Could you check a few things on this model? Use its own coordinates, in mm. Face numbers are marked on the shaded views. A direction names the side the tool comes from. Coordinates: 2 decimals unless noted, no trailing zeros. Order: outer loops, then holes, each group sorted by start corner. A loop starts at its lowest first (then second) coordinate and runs counter-clockwise, first axis right, second up. Notation, with made-up numbers: (40, 3.5) - (85, 3.5) arc R17 ccw to (85, 34.5) - close; hole circle Ø6 at (79, 73). An arc over 180 degrees is marked (long way). Answer as a JSON object with one key per item and string values. Group by question number.
(1) Which directions (+Z, -Z, +X, -X, +Y, -Y) give clear straight access to the entire face, cutting with the end or side of a thin tool? Please do the marked faces 1 and 2.
(2) Imagine slicing it at D-D, the plane x = -15.5. Write out the boundary of the cut face in (y, z).
(3) Imagine slicing it at A-A, the plane z = 1.6. Write out the boundary of the cut face in (x, y).
(4) Will these pins go through, and if not, where does the flat tip stop? P1, Ø10, axis at x = -59, y = 3, coming from the +Z side; P2, Ø1, axis at x = -67.5, z = -0.5, coming from the -Y side; P3, Ø4, axis at x = -10.5, y = 19.5, coming from the -Z side; P4, Ø0.7, axis at y = -52.5, z = 0, coming from the -X side.
(5) Imagine slicing it at B-B, the plane x = 0. Write out the boundary of the cut face in (y, z).
(6) Please list where these lines run through material, in increasing order: probe 1 along Y at (x, z) = (-0.5, 2.45); probe 2 along Y at (x, z) = (-13.5, -0.35); probe 3 along X at (y, z) = (-6.5, -0.65).
(7) Imagine slicing it at C-C, the plane y = -72. Write out the boundary of the cut face in (x, z), and give its area (3 significant figures).
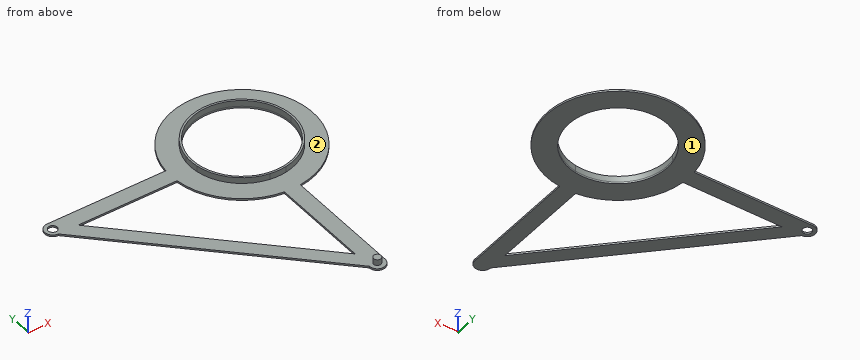
from build123d import *

# Parameters (mm, degrees)
F1_DEPTH = 0.9
F2_DEPTH = 3
F3_DEPTH = 3


with BuildPart() as f1:
    # F0 (on Top) → F1 (new body)
    with BuildSketch(Plane.XY):
        with BuildLine():
            Line((-35.5758344948, 4), (-95.5, 4))
            ThreePointArc((-95.5, 4), (-92.6715728753, 2.8284271247), (-91.5, 0))
            ThreePointArc((-91.5, 0), (-92.6715728753, -2.8284271247), (-95.5, -4))
            Line((-95.5, -4), (-85.6005050634, -4))
            Line((-85.6005050634, -4), (-35.5758344948, -4))
            ThreePointArc((-35.5758344948, -4), (-35.8, 0), (-35.5758344948, 4))
        make_face()
        with BuildLine():
            ThreePointArc((-95.5, 2.25), (-93.9090097423, 1.5909902577), (-93.25, 0))
            ThreePointArc((-93.25, 0), (-93.9090097423, -1.5909902577), (-95.5, -2.25))
            Line((-95.5, -2.25), (-95.5, -4))
            ThreePointArc((-95.5, -4), (-92.6715728753, -2.8284271247), (-91.5, 0))
            ThreePointArc((-91.5, 0), (-92.6715728753, 2.8284271247), (-95.5, 4))
            Line((-95.5, 4), (-95.5, 2.25))
        make_face()
        with BuildLine():
            ThreePointArc((-95.5, -2.25), (-97.75, 0), (-95.5, 2.25))
            Line((-95.5, 2.25), (-95.5, 4))
            ThreePointArc((-95.5, 4), (-99.5, 0), (-95.5, -4))
            Line((-95.5, -4), (-95.5, -2.25))
        make_face()
        Polygon((-85.6005050634, -4), (-95.5, -4), (-4, -95.5), (-4, -85.6005050634), align=None)
        with BuildLine():
            Line((-1.85, -95.5), (-4, -95.5))
            ThreePointArc((-4, -95.5), (0, -99.5), (4, -95.5))
            Line((4, -95.5), (1.85, -95.5))
            ThreePointArc((1.85, -95.5), (0, -97.35), (-1.85, -95.5))
        make_face()
        with BuildLine():
            ThreePointArc((4, -95.5), (0, -91.5), (-4, -95.5))
            Line((-4, -95.5), (-1.85, -95.5))
            ThreePointArc((-1.85, -95.5), (0, -93.65), (1.85, -95.5))
            Line((1.85, -95.5), (4, -95.5))
        make_face()
        with BuildLine():
            Line((1.85, -95.5), (-1.85, -95.5))
            ThreePointArc((-1.85, -95.5), (0, -97.35), (1.85, -95.5))
        make_face()
        with BuildLine():
            ThreePointArc((1.85, -95.5), (0, -93.65), (-1.85, -95.5))
            Line((-1.85, -95.5), (1.85, -95.5))
        make_face()
        with BuildLine():
            Line((-4, -85.6005050634), (-4, -95.5))
            ThreePointArc((-4, -95.5), (0, -91.5), (4, -95.5))
            Line((4, -95.5), (4, -35.5758344948))
            ThreePointArc((4, -35.5758344948), (0, -35.8), (-4, -35.5758344948))
            Line((-4, -35.5758344948), (-4, -85.6005050634))
        make_face()
        with BuildLine():
            Line((-25.4880364093, -4), (-35.5758344948, -4))
            ThreePointArc((-35.5758344948, -4), (-25.3144227665, -25.3144227665), (-4, -35.5758344948))
            Line((-4, -35.5758344948), (-4, -25.4880364093))
            ThreePointArc((-4, -25.4880364093), (-18.2433549546, -18.2433549546), (-25.4880364093, -4))
        make_face()
        with BuildLine():
            Line((-25.4880364093, 4), (-35.5758344948, 4))
            ThreePointArc((-35.5758344948, 4), (-35.8, 0), (-35.5758344948, -4))
            Line((-35.5758344948, -4), (-25.4880364093, -4))
            ThreePointArc((-25.4880364093, -4), (-25.8, 0), (-25.4880364093, 4))
        make_face()
        with BuildLine():
            ThreePointArc((35.8, 0), (2.0031381738, 35.7439146913), (-35.5758344948, 4))
            Line((-35.5758344948, 4), (-25.4880364093, 4))
            ThreePointArc((-25.4880364093, 4), (2.0060733587, 25.7218908652), (25.8, 0))
            ThreePointArc((25.8, 0), (19.6066315312, -16.7696153802), (4, -25.4880364093))
            Line((4, -25.4880364093), (4, -35.5758344948))
            ThreePointArc((4, -35.5758344948), (26.6911970507, -23.858331878), (35.8, 0))
        make_face()
        with BuildLine():
            ThreePointArc((-4, -35.5758344948), (0, -35.8), (4, -35.5758344948))
            Line((4, -35.5758344948), (4, -25.4880364093))
            ThreePointArc((4, -25.4880364093), (0, -25.8), (-4, -25.4880364093))
            Line((-4, -25.4880364093), (-4, -35.5758344948))
        make_face()
        with BuildLine():
            Line((-24.5158234616, -4), (-25.4880364093, -4))
            ThreePointArc((-25.4880364093, -4), (-18.2433549546, -18.2433549546), (-4, -25.4880364093))
            Line((-4, -25.4880364093), (-4, -24.5158234616))
            ThreePointArc((-4, -24.5158234616), (-17.5645324447, -17.5645324447), (-24.5158234616, -4))
        make_face()
        with BuildLine():
            Line((-24.5158234616, 4), (-25.4880364093, 4))
            ThreePointArc((-25.4880364093, 4), (-25.8, 0), (-25.4880364093, -4))
            Line((-25.4880364093, -4), (-24.5158234616, -4))
            ThreePointArc((-24.5158234616, -4), (-24.84, 0), (-24.5158234616, 4))
        make_face()
        with BuildLine():
            ThreePointArc((25.8, 0), (2.0060733587, 25.7218908652), (-25.4880364093, 4))
            Line((-25.4880364093, 4), (-24.5158234616, 4))
            ThreePointArc((-24.5158234616, 4), (2.0065574019, 24.7588232231), (24.84, 0))
            ThreePointArc((24.84, 0), (18.925982141, -16.0882814496), (4, -24.5158234616))
            Line((4, -24.5158234616), (4, -25.4880364093))
            ThreePointArc((4, -25.4880364093), (19.6066315312, -16.7696153802), (25.8, 0))
        make_face()
        with BuildLine():
            ThreePointArc((-4, -25.4880364093), (0, -25.8), (4, -25.4880364093))
            Line((4, -25.4880364093), (4, -24.5158234616))
            ThreePointArc((4, -24.5158234616), (0, -24.84), (-4, -24.5158234616))
            Line((-4, -24.5158234616), (-4, -25.4880364093))
        make_face()
    extrude(amount=-F1_DEPTH)

    # F0 (on Top) → F2 (join)
    with BuildSketch(Plane.XY):
        with BuildLine():
            ThreePointArc((25.8, 0), (2.0060733587, 25.7218908652), (-25.4880364093, 4))
            Line((-25.4880364093, 4), (-24.5158234616, 4))
            ThreePointArc((-24.5158234616, 4), (2.0065574019, 24.7588232231), (24.84, 0))
            ThreePointArc((24.84, 0), (18.925982141, -16.0882814496), (4, -24.5158234616))
            Line((4, -24.5158234616), (4, -25.4880364093))
            ThreePointArc((4, -25.4880364093), (19.6066315312, -16.7696153802), (25.8, 0))
        make_face()
        with BuildLine():
            Line((-24.5158234616, 4), (-25.4880364093, 4))
            ThreePointArc((-25.4880364093, 4), (-25.8, 0), (-25.4880364093, -4))
            Line((-25.4880364093, -4), (-24.5158234616, -4))
            ThreePointArc((-24.5158234616, -4), (-24.84, 0), (-24.5158234616, 4))
        make_face()
        with BuildLine():
            Line((-24.5158234616, -4), (-25.4880364093, -4))
            ThreePointArc((-25.4880364093, -4), (-18.2433549546, -18.2433549546), (-4, -25.4880364093))
            Line((-4, -25.4880364093), (-4, -24.5158234616))
            ThreePointArc((-4, -24.5158234616), (-17.5645324447, -17.5645324447), (-24.5158234616, -4))
        make_face()
        with BuildLine():
            ThreePointArc((-4, -25.4880364093), (0, -25.8), (4, -25.4880364093))
            Line((4, -25.4880364093), (4, -24.5158234616))
            ThreePointArc((4, -24.5158234616), (0, -24.84), (-4, -24.5158234616))
            Line((-4, -24.5158234616), (-4, -25.4880364093))
        make_face()
    extrude(amount=F2_DEPTH)

    # F0 (on Top) → F3 (join)
    with BuildSketch(Plane.XY):
        with BuildLine():
            ThreePointArc((1.85, -95.5), (0, -93.65), (-1.85, -95.5))
            Line((-1.85, -95.5), (1.85, -95.5))
        make_face()
        with BuildLine():
            Line((1.85, -95.5), (-1.85, -95.5))
            ThreePointArc((-1.85, -95.5), (0, -97.35), (1.85, -95.5))
        make_face()
    extrude(amount=F3_DEPTH)


solid = f1.part
Result set:
{
 "1": {"face 1": "-Z, +X, -X, +Y, -Y", "face 2": "+Z"},
 "2": {"outline": "(-84, -0.9) - (-74.1, -0.9) - (-74.1, 0) - (-84, 0) - close; (-32.27, -0.9) - (-19.41, -0.9) - (-19.41, 3) - (-20.62, 3) - (-20.62, 0) - (-32.27, 0) - close; (19.41, -0.9) - (32.27, -0.9) - (32.27, 0) - (20.62, 0) - (20.62, 3) - (19.41, 3) - close"},
 "3": {"outline": "circle Ø51.6 at (0, 0); circle Ø3.7 at (0, -95.5); hole circle Ø49.68 at (0, 0)"},
 "4": {"P1": "stops at z = 0", "P2": "stops at y = -32.5", "P3": "passes through", "P4": "stops at x = -47.35"},
 "5": {"outline": "(-99.5, -0.9) - (-24.84, -0.9) - (-24.84, 3) - (-25.8, 3) - (-25.8, 0) - (-93.65, 0) - (-93.65, 3) - (-97.35, 3) - (-97.35, 0) - (-99.5, 0) - close; (24.84, -0.9) - (35.8, -0.9) - (35.8, 0) - (25.8, 0) - (25.8, 3) - (24.84, 3) - close"},
 "6": {"probe 1": "y = -97.28 to -93.72, -25.8 to -24.83, 24.83 to 25.8", "probe 2": "y = -86 to -76.1, -33.16 to -20.85, 20.85 to 33.16", "probe 3": "x = -93 to -83.1, -35.2 to -23.97, 23.97 to 35.2"},
 "7": {"outline": "(-27.5, -0.9) - (-17.6, -0.9) - (-17.6, 0) - (-27.5, 0) - close; (-4, -0.9) - (4, -0.9) - (4, 0) - (-4, 0) - close", "area": "16.1 mm^2"}
}
